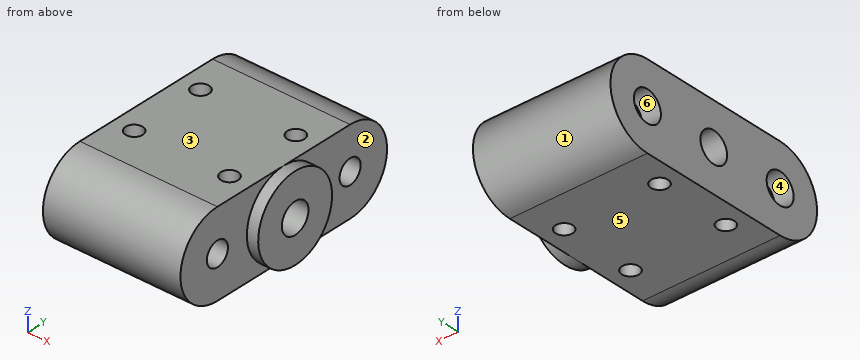
from build123d import *

# Parameters (mm, degrees)
BOSS_EXTRUDE1_DEPTH                  = 23.075011
SKETCH8_R                            = 7.0739
BOSS_EXTRUDE2_DEPTH                  = 1.905
F_1_4_20_TAPPED_HOLE1_D              = 5.1054
F_10_32_TAPPED_HOLE1_D               = 4.0386
F_6_40_TAPPED_HOLE1_D                = 2.8702
F_13_64_0_20313_DIAMETER_HOLE1_D     = 5.159502
F_13_64_0_20313_DIAMETER_HOLE1_DEPTH = 3.175
F_13_64_0_20313_DIAMETER_HOLE1_TIP   = 1.550070783


with BuildPart() as part:
    # Sketch1 → Boss-Extrude1 (new body)
    with BuildSketch(Plane(origin=(0, 0, 0), x_dir=(0, 0, -1), z_dir=(1, 0, 0))):
        with BuildLine():
            Line((7.0739, 12.7), (7.0739, -12.7))
            ThreePointArc((7.0739, -12.7), (0, -19.7739), (-7.0739, -12.7))
            Line((-7.0739, -12.7), (-7.0739, 12.7))
            ThreePointArc((-7.0739, 12.7), (0, 19.7739), (7.0739, 12.7))
        make_face()
    extrude(amount=BOSS_EXTRUDE1_DEPTH)

    # Sketch8 → Boss-Extrude2 (add)
    with BuildSketch(Plane(origin=(23.075011, 0, 0), x_dir=(0, 0, -1), z_dir=(1, 0, 0))):
        Circle(SKETCH8_R)
    extrude(amount=BOSS_EXTRUDE2_DEPTH)

    # 1/4-20 Tapped Hole1 (through all)
    with Locations(Plane(origin=(24.980011, 0, 0), x_dir=(0, 0, -1), z_dir=(1, 0, 0))):
        with Locations((0, 0)):
            Hole(F_1_4_20_TAPPED_HOLE1_D / 2)

    # #10-32 Tapped Hole1 (through all)
    with Locations(Plane(origin=(23.075011, 0, 0), x_dir=(0, 0, -1), z_dir=(1, 0, 0))):
        with Locations((0, 12.7), (0, -12.7)):
            Hole(F_10_32_TAPPED_HOLE1_D / 2)

    # #6-40 Tapped Hole1 (through all)
    with Locations(Plane.XY.offset(7.0739)):
        with Locations((3.5375055, 6.35), (19.5375055, 6.35), (3.5375055, -6.35), (19.5375055, -6.35)):
            Hole(F_6_40_TAPPED_HOLE1_D / 2)

    # 13/64 (0.20313) Diameter Hole1
    with Locations(Plane.ZY):
        with Locations((0, -12.7), (0, 12.7)):
            Hole(F_13_64_0_20313_DIAMETER_HOLE1_D / 2, depth=F_13_64_0_20313_DIAMETER_HOLE1_DEPTH)
            with Locations((0, 0, -(F_13_64_0_20313_DIAMETER_HOLE1_DEPTH + F_13_64_0_20313_DIAMETER_HOLE1_TIP / 2))):  # 118° drill point
                Cone(0, F_13_64_0_20313_DIAMETER_HOLE1_D / 2, F_13_64_0_20313_DIAMETER_HOLE1_TIP, mode=Mode.SUBTRACT)


solid = part.part
Geometry check sheet. Reference: the model listing, model coordinates, mm. Face numbers are marked on the shaded views. A direction names the side the tool comes from. Round coordinates to 2 decimals unless told otherwise and drop trailing zeros. Loops run counter-clockwise (first coordinate to the right, second up) from the corner with the lowest first, then second, coordinate; pieces in that order, holes last. Notation, with made-up numbers: (47.5, 36.5) - (68.5, 36.5) arc R29 ccw to (68.5, 70.5) - close; hole circle Ø6 at (-40, -38.5). An arc over 180 degrees is marked (long way). Answer as CSV lines item,"result".
(1) Depth check by flat-ended pin: pin 1 Ø3 at (x, y) = (17, 14.5) entering from -Z; pin 2 Ø5 at (x, z) = (13.5, 3.5) entering from -Y; pin 3 Ø4.5 at (y, z) = (-12.7, 0) entering from +X (3 decimals). Enter the tip coordinate at first touch or a pass-through.
Output values:
pin 1,"stops at z = -7.07"
pin 2,"stops at y = -19.7"
pin 3,"stops at x = 23.075"
(2) Cross-section at C-C, the plane y = -2. Enter the section's corners in (x, z).
Output values:
outline,"(0, -7.07) - (23.08, -7.07) - (23.08, -6.79) - (24.98, -6.79) - (24.98, -1.59) - (0, -1.59) - close; (0, 1.59) - (24.98, 1.59) - (24.98, 6.79) - (23.08, 6.79) - (23.08, 7.07) - (0, 7.07) - close"
(3) Set-up check for the marked faces 5 and 6: record each of +Z, -Z, +X, -X, +Y, -Y from which the full face is reachable in a straight line by a thin tool's end or side.
Output values:
face 5,"-Z, +X, -X, +Y, -Y"
face 6,"-X"
(4) Material ranges on line 1 along Z through (x, y) = (8.25, -12.7); line 2 along Y through (x, z) = (12.5, 0); line 3 along Y through (x, z) = (5.25, -1.5), recorded low to high.
Output values:
line 1,"z = -7.07 to -2.02, 2.02 to 7.07"
line 2,"y = -19.77 to -14.72, -10.68 to -2.55, 2.55 to 10.68, 14.72 to 19.77"
line 3,"y = -19.61 to -14.05, -11.35 to -2.07, 2.07 to 11.35, 14.05 to 19.61"
(5) Cross-section at B-B, the plane x = 6.25. Enter the section's corners in (y, z), and give its area (3 significant figures).
Output values:
outline,"(-12.7, -7.07) - (12.7, -7.07) arc R7.07 ccw to (12.7, 7.07) - (-12.7, 7.07) arc R7.07 ccw to start; hole circle Ø4.04 at (-12.7, 0); hole circle Ø5.11 at (0, 0); hole circle Ø4.04 at (12.7, 0)"
area,"470 mm²"
(6) Cross-section at D-D, the plane x = 19.25. Enter the section's corners in (y, z), and give its area (3 significant figures).
Output values:
outline,"(-12.7, -7.07) - (-7.76, -7.07) - (-7.76, 7.07) - (-12.7, 7.07) arc R7.07 ccw to start; (-4.94, -7.07) - (4.94, -7.07) - (4.94, 7.07) - (-4.94, 7.07) - close; (7.76, -7.07) - (12.7, -7.07) arc R7.07 ccw to (12.7, 7.07) - (7.76, 7.07) - close; hole circle Ø4.04 at (-12.7, 0); hole circle Ø5.11 at (0, 0); hole circle Ø4.04 at (12.7, 0)"
area,"391 mm²"
(7) Cross-section at A-A, the plane z = 0. Give the number of separate pieces and of enclosed holes in the cut face, and give its area (3 significant figures).
Output values:
separate pieces,"4"
enclosed holes,"4"
area,"592 mm²"
(8) Release check for a two-part mould opening along Z. For the marked faces 1, 2, 3 and 4 record: released by +Z, released by -Z, zero draft, split by the parting line, or undercut.
Output values:
face 1,"split by the parting line"
face 2,"zero draft"
face 3,"released by +Z"
face 4,"undercut"
